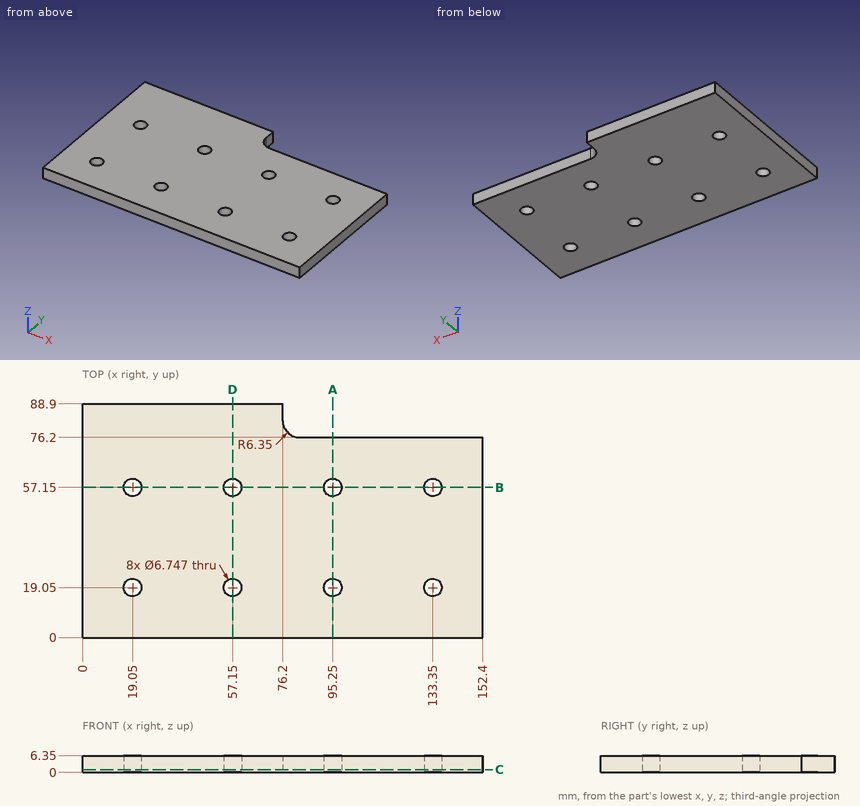
The drawing under review shows one solid part. Ordinate dimensions are in mm from its lowest x, y, z. Round coordinates to 2 decimals unless told otherwise and drop trailing zeros. Loops run counter-clockwise (first coordinate to the right, second up) from the corner with the lowest first, then second, coordinate; pieces in that order, holes last. Notation, with made-up numbers: (-6, 80) - (43, 80) arc R21 ccw to (43, 85) - close; hole circle Ø8 at (-10, 42.25). An arc over 180 degrees is marked (long way). One line per question, with ' | ' between items.
Q1. Take a section at A-A (x = 95.25). Give the boundary of the cut face in (y, z).
Taken from the geometry:
outline: (0, 0) - (15.68, 0) - (15.68, 6.35) - (0, 6.35) - close; (22.42, 0) - (53.78, 0) - (53.78, 6.35) - (22.42, 6.35) - close; (60.52, 0) - (76.2, 0) - (76.2, 6.35) - (60.52, 6.35) - close
Q2. For line 1 along Y through (x, z) = (95.25, 5); line 2 along Y through (x, z) = (19.05, 3.5); line 3 along X through (y, z) = (58.5, 6.25), list the stretches that pass through material, from the lowest coordinate up. Write a range as [from, to].
Taken from the geometry:
line 1: y = [0, 15.68], [22.42, 53.78], [60.52, 76.2] | line 2: y = [0, 15.68], [22.42, 53.78], [60.52, 88.9] | line 3: x = [0, 15.96], [22.14, 54.06], [60.24, 92.16], [98.34, 130.26], [136.44, 152.4]
Q3. Take a section at B-B (y = 57.15). Give the boundary of the cut face in (x, z), and give its area (3 significant figures).
Taken from the geometry:
outline: (0, 0) - (15.68, 0) - (15.68, 6.35) - (0, 6.35) - close; (22.42, 0) - (53.78, 0) - (53.78, 6.35) - (22.42, 6.35) - close; (60.52, 0) - (91.88, 0) - (91.88, 6.35) - (60.52, 6.35) - close; (98.62, 0) - (129.98, 0) - (129.98, 6.35) - (98.62, 6.35) - close; (136.72, 0) - (152.4, 0) - (152.4, 6.35) - (136.72, 6.35) - close | area: 796 mm²
Q4. Take a section at D-D (x = 57.15). Give the boundary of the cut face in (y, z), and give its area (3 significant figures).
Taken from the geometry:
outline: (0, 0) - (15.68, 0) - (15.68, 6.35) - (0, 6.35) - close; (22.42, 0) - (53.78, 0) - (53.78, 6.35) - (22.42, 6.35) - close; (60.52, 0) - (88.9, 0) - (88.9, 6.35) - (60.52, 6.35) - close | area: 479 mm²
Q5. Take a section at C-C (z = 1). State how many separate pieces and enclosed holes the cut face has, and give its area (3 significant figures).
Taken from the geometry:
separate pieces: 1 | enclosed holes: 8 | area: 12,300 mm²
Q6. For pin 1 (11 mm diameter, centred on x = 57.15, y = 19.05, fed in from -Z); pin 2 (6 mm diameter, centred on x = 133.35, y = 57.15, fed in from +Z); pin 3 (3 mm diameter, centred on x = 89.5, z = 3, fed in from +Y), all flat-tipped, find the tip position at first contact; note any pin that passes through.
Taken from the geometry:
pin 1: stops at z = 0 | pin 2: passes through | pin 3: stops at y = 76.2
